Work out the finished part from the listing and answer in its coordinate system (mm). Face numbers are marked on the shaded views. A direction names the side the tool comes from. Coordinates: 2 decimals unless noted, no trailing zeros. Order: outer loops, then holes, each group sorted by start corner. A loop starts at its lowest first (then second) coordinate and runs counter-clockwise, first axis right, second up. Notation, with made-up numbers: (54.5, 7) - (89.5, 7) arc R31 cw to (89.5, 32) - close; hole circle Ø2 at (-3, 44). An arc over 180 degrees is marked (long way). Answer as a JSON object with one key per item and string values. Group by question number.
1) Section A-A (z = -16) is taken. Give the vertices of the cut face in (x, y), plus the area to 3 significant figures.
2) Section B-B (x = 7.5) is taken. Give the vertices of the cut face in (y, z), plus the area to 3 significant figures.
3) The mould has two halves that part along Y. Classify the marked faces 4, 5 and 6: released by +Y, released by -Y, zero draft, split by the parting line, or undercut.
4) Find the intervals of material crossed by line 1 along Y through (x, z) = (-9.5, -2); line 2 along Y through (x, z) = (-25.6, 19.5), in increasing order.
5) Each of these flat-tipped pins is pushed along its axis until it touches: P1, Ø6, axis at x = 17.5, y = -13, coming from the +Z side; P2, Ø1.5, axis at y = 25.5, z = -1.5, coming from the +X side; P3, Ø1, axis at x = -25, z = 4.5, coming from the -Y side; P4, Ø9, axis at y = -13.76, z = 19.5, coming from the -X side. Where does it stop, or does it pass through?
6) A tool of negligible diameter and unlimited length cuts with its end or side. For the marked faces 1, 2 and 3, from which of +Z, -Z, +X, -X, +Y, -Y can it reach the whole face along a straight path? Write none if from no direction.
7) Section C-C (y = 12) is taken. Give the vertices of the cut face in (x, z), plus the area to 3 significant figures.
8) Section D-D (z = 12) is taken. Give the vertices of the cut face in (x, y), plus the area to 3 significant figures.
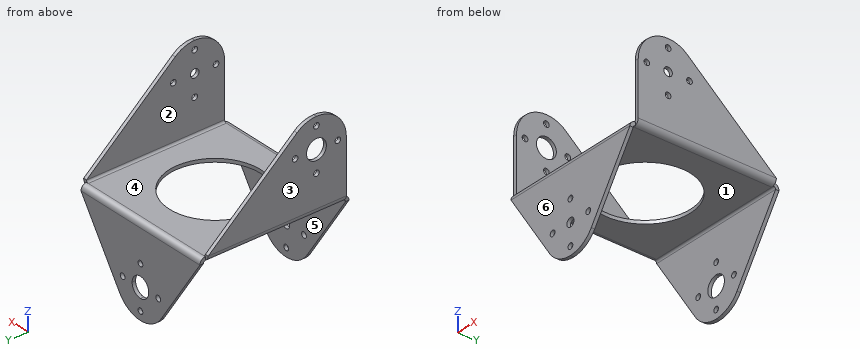
from build123d import *

# Parameters (mm, degrees)
SKETCH_1_W                         = 50
SKETCH_1_H                         = 50
SKETCH_1_R                         = 16
SM_BASE_FLANGE_1_DEPTH             = 1.2
SM_EDGE_FLANGE_1_STRIP_W           = 6.2732
SM_EDGE_FLANGE_1_STRIP_H           = 1.2
SM_EDGE_FLANGE_1_STRIP_CUT_DEPTH   = 50
SM_EDGE_FLANGE_1_STRIP_2_W         = 6.2732
SM_EDGE_FLANGE_1_STRIP_2_H         = 1.2
SM_EDGE_FLANGE_1_STRIP_CUT_2_DEPTH = 50
SM_EDGE_FLANGE_1_DEPTH             = 50
SM_EDGE_FLANGE_1_BEND_DEPTH        = 50
SM_EDGE_FLANGE_2_STRIP_W           = 6.2732
SM_EDGE_FLANGE_2_STRIP_H           = 1.2
SM_EDGE_FLANGE_2_STRIP_CUT_DEPTH   = 48.5268
SM_EDGE_FLANGE_2_STRIP_2_W         = 6.2732
SM_EDGE_FLANGE_2_STRIP_2_H         = 1.2
SM_EDGE_FLANGE_2_STRIP_CUT_2_DEPTH = 48.5268
SM_EDGE_FLANGE_2_DEPTH             = 48.5268
SM_EDGE_FLANGE_2_BEND_DEPTH        = 48.5268
SKETCH_23_R                        = 1
CUT_EXTRUDE_1_DEPTH                = 98
EXTRUDE_START                      = -1.2
SKETCH_30_R                        = 3.5
SKETCH_30_R_2                      = 1.5
EXTRUDE_1_DEPTH                    = 1.2
SKETCH_40_R                        = 1
CUT_EXTRUDE_2_DEPTH                = 67.374995292
SKETCH_40_3_R                      = 1.5
CUT_EXTRUDE_3_DEPTH                = 10
SKETCH_45_R                        = 3.5
CUT_EXTRUDE_4_DEPTH                = 10


# Sheet-metal steps are written as plain solids
with BuildPart() as part:
    # Sketch 1 → 基材-凸緣1 (new body)
    with BuildSketch(Plane.XY):
        Rectangle(SKETCH_1_W, SKETCH_1_H)
        Circle(SKETCH_1_R, mode=Mode.SUBTRACT)
    extrude(amount=-SM_BASE_FLANGE_1_DEPTH)

    # 邊線-凸緣1 strip (across the edge) → 邊線-凸緣1 strip cut (cut)
    with BuildSketch(Plane(origin=(-25, 25, -1.2), x_dir=(0, -1, 0), z_dir=(1, 0, 0))):
        with Locations((-2.4, -0.6)):
            Rectangle(SM_EDGE_FLANGE_1_STRIP_W, SM_EDGE_FLANGE_1_STRIP_H)
    extrude(amount=SM_EDGE_FLANGE_1_STRIP_CUT_DEPTH, mode=Mode.SUBTRACT)

    # 邊線-凸緣1 strip 2 (across the edge) → 邊線-凸緣1 strip cut 2 (cut)
    with BuildSketch(Plane(origin=(25, -25, -1.2), x_dir=(0, 1, 0), z_dir=(-1, 0, 0))):
        with Locations((-2.4, -0.6)):
            Rectangle(SM_EDGE_FLANGE_1_STRIP_2_W, SM_EDGE_FLANGE_1_STRIP_2_H)
    extrude(amount=SM_EDGE_FLANGE_1_STRIP_CUT_2_DEPTH, mode=Mode.SUBTRACT)

    # 邊線-凸緣1 section (across the edge) → 邊線-凸緣1 (add)
    with BuildSketch(Plane(origin=(-25, 25, -1.2), x_dir=(0, -1, 0), z_dir=(1, 0, 0))):
        with BuildLine():
            Line((-1.2, 0.7366), (-1.2, 30))
            Line((-1.2, 30), (0, 30))
            Line((0, 30), (0, 0.7366))
            ThreePointArc((0, 0.7366), (0.215745145, 0.215745145), (0.7366, 0))
            Line((0.7366, 0), (0.7366, -1.2))
            ThreePointArc((0.7366, -1.2), (-0.632782992, -0.632782992), (-1.2, 0.7366))
        make_face()
    extrude(amount=SM_EDGE_FLANGE_1_DEPTH)

    # 邊線-凸緣1 section 2 (across the edge) → 邊線-凸緣1 bend (add)
    with BuildSketch(Plane(origin=(25, -25, -1.2), x_dir=(0, 1, 0), z_dir=(-1, 0, 0))):
        with BuildLine():
            Line((-1.2, 0.7366), (-1.2, 30))
            Line((-1.2, 30), (0, 30))
            Line((0, 30), (0, 0.7366))
            ThreePointArc((0, 0.7366), (0.215745145, 0.215745145), (0.7366, 0))
            Line((0.7366, 0), (0.7366, -1.2))
            ThreePointArc((0.7366, -1.2), (-0.632782992, -0.632782992), (-1.2, 0.7366))
        make_face()
    extrude(amount=SM_EDGE_FLANGE_1_BEND_DEPTH)

    # 邊線-凸緣2 strip (across the edge) → 邊線-凸緣2 strip cut (cut)
    with BuildSketch(Plane(origin=(25, -24.2634, 0), x_dir=(-1, 0, 0), z_dir=(0, 1, 0))):
        with Locations((-2.4, -0.6)):
            Rectangle(SM_EDGE_FLANGE_2_STRIP_W, SM_EDGE_FLANGE_2_STRIP_H)
    extrude(amount=SM_EDGE_FLANGE_2_STRIP_CUT_DEPTH, mode=Mode.SUBTRACT)

    # 邊線-凸緣2 strip 2 (across the edge) → 邊線-凸緣2 strip cut 2 (cut)
    with BuildSketch(Plane(origin=(-25, 24.2634, 0), x_dir=(1, 0, 0), z_dir=(0, -1, 0))):
        with Locations((-2.4, -0.6)):
            Rectangle(SM_EDGE_FLANGE_2_STRIP_2_W, SM_EDGE_FLANGE_2_STRIP_2_H)
    extrude(amount=SM_EDGE_FLANGE_2_STRIP_CUT_2_DEPTH, mode=Mode.SUBTRACT)

    # 邊線-凸緣2 section (across the edge) → 邊線-凸緣2 (add)
    with BuildSketch(Plane(origin=(25, -24.2634, 0), x_dir=(-1, 0, 0), z_dir=(0, 1, 0))):
        with BuildLine():
            Line((-1.2, 0.7366), (-1.2, 30))
            Line((-1.2, 30), (0, 30))
            Line((0, 30), (0, 0.7366))
            ThreePointArc((0, 0.7366), (0.215745145, 0.215745145), (0.7366, 0))
            Line((0.7366, 0), (0.7366, -1.2))
            ThreePointArc((0.7366, -1.2), (-0.632782992, -0.632782992), (-1.2, 0.7366))
        make_face()
    extrude(amount=SM_EDGE_FLANGE_2_DEPTH)

    # 邊線-凸緣2 section 2 (across the edge) → 邊線-凸緣2 bend (add)
    with BuildSketch(Plane(origin=(-25, 24.2634, 0), x_dir=(1, 0, 0), z_dir=(0, -1, 0))):
        with BuildLine():
            Line((-1.2, 0.7366), (-1.2, 30))
            Line((-1.2, 30), (0, 30))
            Line((0, 30), (0, 0.7366))
            ThreePointArc((0, 0.7366), (0.215745145, 0.215745145), (0.7366, 0))
            Line((0.7366, 0), (0.7366, -1.2))
            ThreePointArc((0.7366, -1.2), (-0.632782992, -0.632782992), (-1.2, 0.7366))
        make_face()
    extrude(amount=SM_EDGE_FLANGE_2_BEND_DEPTH)

    # 草圖23 → 除料-伸長1 (cut)
    with BuildSketch(Plane(origin=(0, 26.2, 0), x_dir=(1, 0, 0), z_dir=(0, 1, 0))):
        with BuildLine():
            Line((25, 31.2), (0, 31.2))
            ThreePointArc((0, 31.2), (4.971280899, 29.948587256), (8.757585745, 26.492641186))
            Line((8.757585745, 26.492641186), (25, 1.9366))
            Line((25, 1.9366), (25, 31.2))
        make_face()
        with BuildLine():
            ThreePointArc((-8.757585745, 26.492641186), (-4.971280899, 29.948587256), (0, 31.2))
            Line((0, 31.2), (-25, 31.2))
            Line((-25, 31.2), (-25, 1.9366))
            Line((-25, 1.9366), (-8.757585745, 26.492641186))
        make_face()
        with BuildLine():
            ThreePointArc((1, 28.2), (0.707106781, 28.907106781), (0, 29.2))
            Line((0, 29.2), (0, 27.2))
            ThreePointArc((0, 27.2), (0.707106781, 27.492893219), (1, 28.2))
        make_face()
        with BuildLine():
            Line((0, 27.2), (0, 29.2))
            ThreePointArc((0, 29.2), (-1, 28.2), (0, 27.2))
        make_face()
        with Locations(Location((-7.5, 20.7, 0), (0, 0, 90))):
            Circle(SKETCH_23_R)
        with Locations(Location((7.5, 20.7, 0), (0, 0, 90))):
            Circle(SKETCH_23_R)
        with BuildLine():
            ThreePointArc((1, 13.2), (0.707106781, 13.907106781), (0, 14.2))
            Line((0, 14.2), (0, 12.2))
            ThreePointArc((0, 12.2), (0.707106781, 12.492893219), (1, 13.2))
        make_face()
        with BuildLine():
            Line((0, 12.2), (0, 14.2))
            ThreePointArc((0, 14.2), (-1, 13.2), (0, 12.2))
        make_face()
        with BuildLine():
            ThreePointArc((3.5, 20.7), (2.474873734, 23.174873734), (0, 24.2))
            Line((0, 24.2), (0, 17.2))
            ThreePointArc((0, 17.2), (2.474873734, 18.225126266), (3.5, 20.7))
        make_face()
        with BuildLine():
            Line((0, 17.2), (0, 24.2))
            ThreePointArc((0, 24.2), (-3.5, 20.7), (0, 17.2))
        make_face()
    extrude(amount=-CUT_EXTRUDE_1_DEPTH, mode=Mode.SUBTRACT)

    # 草圖30 → 填料-伸長1 (add)
    with BuildSketch(Plane.XZ.offset(26.2).offset(EXTRUDE_START)):
        with Locations(Location((0, -20.7, 0), (0, 0, 270))):
            Circle(SKETCH_30_R)
        with Locations(Location((0, -20.7, 0), (0, 0, 270))):
            Circle(SKETCH_30_R_2, mode=Mode.SUBTRACT)
    extrude(amount=EXTRUDE_1_DEPTH)

    # 草圖40 → 除料-伸長2 (cut, through all)
    with BuildSketch(Plane(origin=(26.2, 0, 0), x_dir=(0, 0, -1), z_dir=(1, 0, 0))):
        with BuildLine():
            Line((-27.472406899, -6.93033859), (-0.7366, 24.2634))
            Line((-0.7366, 24.2634), (-30, 24.2634))
            Line((-30, 24.2634), (-30, -13.763399983))
            ThreePointArc((-30, -13.763399983), (-29.347849317, -10.12061757), (-27.472406899, -6.93033859))
        make_face()
        with BuildLine():
            ThreePointArc((-19.5, -24.2634), (-26.924621208, -21.188021196), (-30, -13.763399983))
            Line((-30, -13.763399983), (-30, -24.2634))
            Line((-30, -24.2634), (-19.5, -24.2634))
        make_face()
        with Locations(Location((-19.5, -6.2634, 0), (0, 0, 180))):
            Circle(SKETCH_40_R)
        with Locations(Location((-12, -13.7634, 0), (0, 0, 180))):
            Circle(SKETCH_40_R)
        with Locations(Location((-19.5, -21.2634, 0), (0, 0, 180))):
            Circle(SKETCH_40_R)
        with Locations(Location((-27, -13.7634, 0), (0, 0, 180))):
            Circle(SKETCH_40_R)
    extrude(amount=-CUT_EXTRUDE_2_DEPTH, mode=Mode.SUBTRACT)

    # 草圖40<3> → 除料-伸長3 (cut)
    with BuildSketch(Plane(origin=(26.2, 0, 0), x_dir=(0, 0, -1), z_dir=(1, 0, 0))):
        with Locations((-19.5, -13.7634)):
            Circle(SKETCH_40_3_R)
    extrude(amount=-CUT_EXTRUDE_3_DEPTH, mode=Mode.SUBTRACT)

    # 草圖45 → 除料-伸長4 (cut)
    with BuildSketch(Plane.ZY.offset(26.2)):
        with Locations((19.5, -13.7634)):
            Circle(SKETCH_45_R)
    extrude(amount=-CUT_EXTRUDE_4_DEPTH, mode=Mode.SUBTRACT)


solid = part.part
Report:
{
 "1": {"outline": "(-15.7, -26.2) - (15.7, -26.2) - (15.7, -25) - (-15.7, -25) - close; (-15.7, 25) - (15.7, 25) - (15.7, 26.2) - (-15.7, 26.2) - close", "area": "75.3 mm²"},
 "2": {"outline": "(-26.2, -28.05) - (-25, -28.05) - (-25, -21.7) - (-26.2, -21.7) - close; (-26.2, -19.7) - (-25, -19.7) - (-25, -1.94) arc R0.74 cw to (-24.26, -1.2) - (-14.13, -1.2) - (-14.13, 0) - (-24.26, 0) arc R1.94 ccw to (-26.2, -1.94) - close; (14.13, -1.2) - (24.26, -1.2) arc R0.74 cw to (25, -1.94) - (25, -19.7) - (26.2, -19.7) - (26.2, -1.94) arc R1.94 ccw to (24.26, 0) - (14.13, 0) - close; (25, -28.05) - (26.2, -28.05) - (26.2, -21.7) - (25, -21.7) - close", "area": "87.2 mm²"},
 "3": {"face 4": "zero draft", "face 5": "undercut", "face 6": "released by -Y"},
 "4": {"line 1": "y = -26.2 to -25, 25 to 26.2", "line 2": "y = -24.26 to -22.26, -20.26 to -17.26, -10.26 to -7.26, -5.26 to 2.37"},
 "5": {"P1": "stops at z = 0", "P2": "stops at x = 25", "P3": "stops at y = -24.26", "P4": "stops at x = -26.2"},
 "6": {"face 1": "-Z, +X, -X", "face 2": "+Z, +Y, -Y", "face 3": "+Z, -Z, -X, +Y, -Y"},
 "7": {"outline": "(-26.2, 0.74) arc R1.94 ccw to (-24.26, -1.2) - (-10.58, -1.2) - (-10.58, 0) - (-24.26, 0) arc R0.74 cw to (-25, 0.74) - (-25, 11.25) - (-26.2, 11.25) - close; (10.58, -1.2) - (24.26, -1.2) arc R1.94 ccw to (26.2, 0.74) - (26.2, 11.25) - (25, 11.25) - (25, 0.74) arc R0.74 cw to (24.26, 0) - (10.58, 0) - close", "area": "63.1 mm²"},
 "8": {"outline": "(-26.2, -24.26) - (-25, -24.26) - (-25, -14.76) - (-26.2, -14.76) - close; (-26.2, -12.76) - (-25, -12.76) - (-25, 11.12) - (-26.2, 11.12) - close; (25, -24.26) - (26.2, -24.26) - (26.2, -14.76) - (25, -14.76) - close; (25, -12.76) - (26.2, -12.76) - (26.2, 11.12) - (25, 11.12) - close", "area": "80.1 mm²"}
}
